from build123d import *

# Parameters (mm, degrees)
SKETCH1_W           = 241.3
SKETCH1_H           = 198.12
BOSS_EXTRUDE1_DEPTH = 5.334
SKETCH2_W           = 5.334
SKETCH2_H           = 9.652
SKETCH2_H_2         = 96.012
SKETCH2_H_3         = 53.848
CUT_EXTRUDE1_DEPTH  = 179.277190048
SKETCH3_W           = 5.334
SKETCH3_H           = 16.256
SKETCH3_H_2         = 130.048
CUT_EXTRUDE2_DEPTH  = 179.277190048
CUT_EXTRUDE5_DEPTH  = 179.277190048
CUT_EXTRUDE6_DEPTH  = 179.277190048
CUT_EXTRUDE7_DEPTH  = 179.277190048
SKETCH8_R           = 0.889
CUT_EXTRUDE8_DEPTH  = 179.277190048
SKETCH9_R           = 0.889
CUT_EXTRUDE9_DEPTH  = 179.277190048


with BuildPart() as part:
    # Sketch1 → Boss-Extrude1 (new body)
    with BuildSketch(Plane.XY):
        with Locations((-21.329797884, -8.624919689)):
            Rectangle(SKETCH1_W, SKETCH1_H)
    extrude(amount=BOSS_EXTRUDE1_DEPTH)

    # Sketch2 → Cut-Extrude1 (cut, through all)
    with BuildSketch(Plane.XY.offset(5.334)):
        with Locations((96.653202116, -102.858919689)):
            Rectangle(SKETCH2_W, SKETCH2_H)
        with Locations((96.653202116, -30.722919689)):
            Rectangle(SKETCH2_W, SKETCH2_H_2)
        with Locations((96.653202116, 63.511080311)):
            Rectangle(SKETCH2_W, SKETCH2_H_3)
    extrude(amount=-CUT_EXTRUDE1_DEPTH, mode=Mode.SUBTRACT)

    # Sketch3 → Cut-Extrude2 (cut, through all)
    with BuildSketch(Plane.XY.offset(5.334)):
        with Locations((-139.312797884, -99.556919689)):
            Rectangle(SKETCH3_W, SKETCH3_H)
        with Locations((-139.312797884, -0.496919689)):
            Rectangle(SKETCH3_W, SKETCH3_H_2)
    extrude(amount=-CUT_EXTRUDE2_DEPTH, mode=Mode.SUBTRACT)

    # Sketch5 → Cut-Extrude5 (cut, through all)
    with BuildSketch(Plane.XY.offset(5.334)):
        Polygon((-136.645797884, -91.428919689), (93.986202116, -107.684919689), (93.986202116, -162.860416997), (-136.645797884, -146.604416997), align=None)
    extrude(amount=-CUT_EXTRUDE5_DEPTH, mode=Mode.SUBTRACT)

    # Sketch6 → Cut-Extrude6 (cut, through all)
    with BuildSketch(Plane.XY.offset(5.334)):
        Polygon((-136.645797884, 90.435080311), (93.986202116, 46.239080311), (93.986202116, 90.435080311), (-136.645797884, 134.631080311), align=None)
    extrude(amount=-CUT_EXTRUDE6_DEPTH, mode=Mode.SUBTRACT)

    # Sketch7 → Cut-Extrude7 (cut, through all)
    with BuildSketch(Plane.XY.offset(5.334)):
        with BuildLine():
            Line((-131.85688859, 89.517381834), (93.986202116, 46.239080311))
            ThreePointArc((93.986202116, 46.239080311), (33.516562096, 36.909943164), (-21.329797884, 9.790080311))
            ThreePointArc((-21.329797884, 9.790080311), (-67.77177066, 61.883202454), (-131.85688859, 89.517381834))
        make_face()
        with BuildLine():
            Line((-136.645797884, -91.428919689), (93.309245371, -107.637204677))
            ThreePointArc((93.309245371, -107.637204677), (28.257929174, -87.626903784), (-21.329797884, -41.009919689))
            ThreePointArc((-21.329797884, -41.009919689), (-73.717554191, -78.2732768), (-136.645797884, -91.428919689))
        make_face()
        with BuildLine():
            ThreePointArc((93.986202116, 7.631080311), (47.550679246, 1.726898301), (4.070202116, -15.609919689))
            ThreePointArc((4.070202116, -15.609919689), (41.092439587, -54.093369858), (92.347831876, -69.076919689))
            ThreePointArc((92.347831876, -69.076919689), (131.631647498, -31.544467715), (93.986202116, 7.631080311))
        make_face()
        with BuildLine():
            ThreePointArc((-136.645797884, 51.573080311), (-81.408536453, 33.982932584), (-46.514432981, -12.3092902))
            ThreePointArc((-46.514432981, -12.3092902), (-87.289086913, -42.04513502), (-136.645797884, -52.566919689))
            ThreePointArc((-136.645797884, -52.566919689), (-188.715797884, -0.496919689), (-136.645797884, 51.573080311))
        make_face()
    extrude(amount=-CUT_EXTRUDE7_DEPTH, mode=Mode.SUBTRACT)

    # Sketch8 → Cut-Extrude8 (cut, through all)
    with BuildSketch(Plane.XY.offset(5.334)):
        with Locations((-130.295797884, 77.481080311)):
            Circle(SKETCH8_R)
        with Locations(Location((-130.295797884, -78.474919689, 0), (0, 0, 180))):
            Circle(SKETCH8_R)
    extrude(amount=-CUT_EXTRUDE8_DEPTH, mode=Mode.SUBTRACT)

    # Sketch9 → Cut-Extrude9 (cut, through all)
    with BuildSketch(Plane.XY.offset(5.334)):
        with Locations((87.636202116, 26.935080311)):
            Circle(SKETCH9_R)
        with Locations(Location((87.636202116, -88.380919689, 0), (0, 0, 180))):
            Circle(SKETCH9_R)
    extrude(amount=-CUT_EXTRUDE9_DEPTH, mode=Mode.SUBTRACT)


solid = part.part
Design review of the part built by this model. Coordinates are the model's own, in mm. A direction names the side the tool comes from. Give positions to 0.01 mm unless a question says otherwise; leave off trailing zeros. Order: outer loops, then holes, each group sorted by start corner. A loop starts at its lowest first (then second) coordinate and runs counter-clockwise, first axis right, second up.
1. For pin 1 Ø2 at (y, z) = (56.5, 3.5) entering from -X; pin 2 Ø1.6 at (y, z) = (12, 3) entering from +X; pin 3 Ø2 at (x, y) = (-130.3, 77.48) entering from +Z; pin 4 Ø2 at (x, z) = (39, 4) entering from -Y, all flat-tipped, find the tip position at first contact; note any pin that passes through.
Solution:
pin 1: stops at x = -136.65
pin 2: stops at x = 93.99
pin 3: stops at z = 5.33
pin 4: stops at y = -93.78
2. Add section A-A, the plane x = 27.5. State the section outline as (y, z) points.
Solution:
outline: (-87.18, 0) - (-44.28, 0) - (-44.28, 5.33) - (-87.18, 5.33) - close; (-4.69, 0) - (34.9, 0) - (34.9, 5.33) - (-4.69, 5.33) - close
3. Add section C-C, the plane x = -74.5. State the section outline as (y, z) points.
Solution:
outline: (-78.61, 0) - (-35.39, 0) - (-35.39, 5.33) - (-78.61, 5.33) - close; (28.59, 0) - (66.48, 0) - (66.48, 5.33) - (28.59, 5.33) - close
4. To check wall thickness, follow L1, parallel to Y at x = -101, z = 2.8; L2, parallel to Y at x = -127.5, z = 0.45; L3, parallel to X at y = 28.5, z = 2.1. State the ranges of each line that lie inside material, in increasing order.
Solution:
L1: y = -87.33 to -47.2, 44.67 to 80.34
L2: y = -91.16 to -52.22, 51.13 to 88.62
L3: x = -74.39 to -33.58, 11.5 to 99.32
5. Add section D-D, the plane y = -19. State the section outline as (x, z) points.
Solution:
outline: (-52.99, 0) - (6.03, 0) - (6.03, 5.33) - (-52.99, 5.33) - close
6. Tool access review of faces 1 (the flat face through (97, -78.729, 3)), 2 (the flat face through (97, -98.033, 3)), 3 (the flat face through (-136.646, 58, 3)), 4 (the cylindrical face through (34.34, 37.17, 2.7)): name each direction out of +Z, -Z, +X, -X, +Y, -Y from which nothing blocks a thin tool from reaching the whole face with its end or side.
Solution:
face 1: +Z, -Z, +X
face 2: +Z, -Z, +X, -Y
face 3: +Z, -Z, -X
face 4: +Z, -Z, +Y
7. Add section B-B, the plane z = 4. State how many separate pieces and enclosed holes the cut face has, then the cut area to 3 significant figures.
Solution:
separate pieces: 1
enclosed holes: 4
area: 18,900 mm2
